```python
from build123d import *

# Parameters (mm, degrees)
ESBO_O1_R                 = 12.5
RESSALTO_EXTRUS_O2_DEPTH  = 21
ESBO_O2_R                 = 12.2
RESSALTO_EXTRUS_O3_DEPTH  = 31
ESBO_O3_R                 = 3.5
RESSALTO_EXTRUS_O4_DEPTH  = 2
ESBO_O4_R                 = 2
RESSALTO_EXTRUS_O6_DEPTH  = 10
CORTE_EXTRUS_O1_DEPTH     = 8
ESBO_O7_R                 = 12.2
RESSALTO_EXTRUS_O8_DEPTH  = 1.5
ESBO_O8_R                 = 0.75
RESSALTO_EXTRUS_O9_DEPTH  = 1
ESBO_O9_R                 = 7
RESSALTO_EXTRUS_O10_DEPTH = 3


with BuildPart() as part:
    # Esboço1 → Ressalto-extrusão2 (new body)
    with BuildSketch(Plane.XY):
        with Locations(Location((0, 0, 0), (0, 0, 180))):
            Circle(ESBO_O1_R)
    extrude(amount=RESSALTO_EXTRUS_O2_DEPTH)

    # Esboço2 → Ressalto-extrusão3 (add)
    with BuildSketch(Plane(origin=(0, 0, 0), x_dir=(-1, 0, 0), z_dir=(0, 0, -1))):
        Circle(ESBO_O2_R)
    extrude(amount=RESSALTO_EXTRUS_O3_DEPTH)

    # Esboço3 → Ressalto-extrusão4 (add)
    with BuildSketch(Plane.XY.offset(21)):
        Circle(ESBO_O3_R)
    extrude(amount=RESSALTO_EXTRUS_O4_DEPTH)

    # Esboço4 → Ressalto-extrusão6 (add)
    with BuildSketch(Plane.XY.offset(23)):
        Circle(ESBO_O4_R)
    extrude(amount=RESSALTO_EXTRUS_O6_DEPTH)

    # Esboço6 → Corte-extrusão1 (cut)
    with BuildSketch(Plane.XY.offset(33)):
        Polygon((0, 2), (3.689966046, 2), (3.689966046, 1), (-3.825112122, 1), (-3.825112122, 2), align=None)
    extrude(amount=-CORTE_EXTRUS_O1_DEPTH, mode=Mode.SUBTRACT)

    # Esboço7 → Ressalto-extrusão8 (add)
    with BuildSketch(Plane(origin=(0, 0, -31), x_dir=(-1, 0, 0), z_dir=(0, 0, -1))):
        Circle(ESBO_O7_R)
    extrude(amount=RESSALTO_EXTRUS_O8_DEPTH)

    # Esboço8 → Ressalto-extrusão9 (add)
    with BuildSketch(Plane(origin=(0, 0, -32.5), x_dir=(-1, 0, 0), z_dir=(0, 0, -1))):
        Circle(ESBO_O8_R)
    extrude(amount=RESSALTO_EXTRUS_O9_DEPTH)

    # Esboço9 → Ressalto-extrusão10 (add)
    with BuildSketch(Plane(origin=(0, 0, -33.5), x_dir=(-1, 0, 0), z_dir=(0, 0, -1))):
        Circle(ESBO_O9_R)
    extrude(amount=RESSALTO_EXTRUS_O10_DEPTH)


solid = part.part
```
Build history of the part. All positions in model axes, mm. A direction names the side the tool comes from. Round coordinates to 2 decimals unless told otherwise and drop trailing zeros. Write each loop counter-clockwise with the first axis right and the second up, starting at its lowest first coordinate (ties: lowest second). Pieces come first, ordered by that corner, then holes.
1) 3-axis set-ups, long thin cutter, end or side, ignore diameter. For faces 1 (the cylindrical face through (3.233, -1.341, 21.986)), 2 (the flat face through (0, 0, -36.5)), 3 (the cylindrical face through (-6.466, -2.681, -34.979)): which of +Z, -Z, +X, -X, +Y, -Y reach the whole face in a straight line?
2) Pin check, flat tips, straight feed: pin 1 (0.5 mm diameter, centred on x = -1, y = 1.5, fed in from +Z); pin 2 (4 mm diameter, centred on x = 0, z = 30, fed in from +Y); pin 3 (12 mm diameter, centred on x = -8, y = 3, fed in from +Z); pin 4 (10 mm diameter, centred on x = -4, z = 4.5, fed in from +Y). Stop position of each tip, or through.
3) Band-saw the part on D-D, the plane z = -2.5. List the corners of the cut face in (x, y), and give its area (3 significant figures).
4) Band-saw the part on C-C, the plane x = 4.5. List the corners of the cut face in (y, z), and give its area (3 significant figures).
5) Mould opens along Z. For faces 4 (the cylindrical face through (0.75, 0.03, -32.99)), 5 (the flat face through (2, -2, 23)), 6 (the flat face through (0, 1, 29)) say: +Z half, -Z half, draft (parallel to the pull), parting line (faces both ways), or undercut.
6) Drill centre lines: probe 1 along Z at (x, y) = (2.5, 0.5); probe 2 along Z at (x, y) = (4.75, -3.5); probe 3 along Z at (x, y) = (7.25, -6.75). Where is each one in solid material? Low to high.
7) Band-saw the part on A-A, the plane x = 0. List the corners of the cut face in (y, z), and give its area (3 significant figures).
8) Band-saw the part on B-B, the plane y = 0. List the corners of the cut face in (x, z), and give its area (3 significant figures).
Ans:
1. face 1: +Z
1. face 2: -Z, +X, -X, +Y, -Y
1. face 3: -Z
2. pin 1: stops at z = 25
2. pin 2: stops at y = 1
2. pin 3: stops at z = 23
2. pin 4: stops at y = 12.5
3. outline: circle Ø24.4 at (0, 0)
3. area: 468 mm2
4. outline: (-11.66, 0) - (-11.34, 0) - (-11.34, -32.5) - (11.34, -32.5) - (11.34, 0) - (11.66, 0) - (11.66, 21) - (-11.66, 21) - close; (-5.36, -36.5) - (5.36, -36.5) - (5.36, -33.5) - (-5.36, -33.5) - close
4. area: 1,260 mm2
5. face 4: undercut
5. face 5: +Z half
5. face 6: draft
6. probe 1: z = -36.5 to -33.5, -32.5 to 23
6. probe 2: z = -36.5 to -33.5, -32.5 to 21
6. probe 3: z = -32.5 to 21
7. outline: (-12.5, 0) - (-12.2, 0) - (-12.2, -32.5) - (-0.75, -32.5) - (-0.75, -33.5) - (-7, -33.5) - (-7, -36.5) - (7, -36.5) - (7, -33.5) - (0.75, -33.5) - (0.75, -32.5) - (12.2, -32.5) - (12.2, 0) - (12.5, 0) - (12.5, 21) - (3.5, 21) - (3.5, 23) - (2, 23) - (2, 25) - (1, 25) - (1, 33) - (-2, 33) - (-2, 23) - (-3.5, 23) - (-3.5, 21) - (-12.5, 21) - close
7. area: 1,410 mm2
8. outline: (-12.5, 0) - (-12.2, 0) - (-12.2, -32.5) - (-0.75, -32.5) - (-0.75, -33.5) - (-7, -33.5) - (-7, -36.5) - (7, -36.5) - (7, -33.5) - (0.75, -33.5) - (0.75, -32.5) - (12.2, -32.5) - (12.2, 0) - (12.5, 0) - (12.5, 21) - (3.5, 21) - (3.5, 23) - (2, 23) - (2, 33) - (-2, 33) - (-2, 23) - (-3.5, 23) - (-3.5, 21) - (-12.5, 21) - close
8. area: 1,420 mm2
